```python
from build123d import *

# Parameters (mm, degrees)
F0_W     = 10
F0_H     = 20
F0_W_2   = 5
F1_DEPTH = 2.5


with BuildPart() as f1:
    # F0 (on Front) → F1 (new body, symmetric)
    with BuildSketch(Plane.XZ):
        Polygon((-42.5, -5), (42.5, -5), (42.5, 5), (32.5, 5), (27.5, 5), (22.5, 5), (17.5, 5), (12.5, 5), (7.5, 5), (2.5, 5), (-2.5, 5), (-7.5, 5), (-12.5, 5), (-17.5, 5), (-22.5, 5), (-27.5, 5), (-32.5, 5), (-42.5, 5), align=None)
        with Locations((37.5, 15)):
            Rectangle(F0_W, F0_H)
        with Locations((-37.5, 15)):
            Rectangle(F0_W, F0_H)
        with Locations((25, 15)):
            Rectangle(F0_W_2, F0_H)
        with Locations((-25, 15)):
            Rectangle(F0_W_2, F0_H)
        with Locations((15, 15)):
            Rectangle(F0_W_2, F0_H)
        with Locations((-15, 15)):
            Rectangle(F0_W_2, F0_H)
        with Locations((5, 15)):
            Rectangle(F0_W_2, F0_H)
        with Locations((-5, 15)):
            Rectangle(F0_W_2, F0_H)
    extrude(amount=F1_DEPTH, both=True)


solid = f1.part
```
Geometry: final body of the model. Coordinates: model frame, mm. A direction names the side the tool comes from. Round coordinates to 2 decimals unless told otherwise and drop trailing zeros. Loops run counter-clockwise (first coordinate to the right, second up) from the corner with the lowest first, then second, coordinate; pieces in that order, holes last. Notation, with made-up numbers: (23, -16) -> (59, -16) arc R20 ccw to (59, 12) -> close; hole circle Ø7 at (31, -33). An arc over 180 degrees is marked (long way). Write each question's results on one line, items separated by ' | '.
Item 1: Pull-direction query (X, two-part tool) for faces 1 (the face through (-42.5, 0, 10)), 2 (the face through (-1, -2.5, 4)), 3 (the face through (-27.5, 0, 15)); classes: pulls with the +X half, pulls with the -X half, needs draft (parallel to the pull), parting line crosses it, or undercut.
Answers below:
face 1: pulls with the -X half | face 2: needs draft | face 3: undercut
Item 2: Pin query (flat end, axial travel): pin 1 Ø5 at (x, z) = (-29, 7) entering from +Y; pin 2 Ø2 at (x, y) = (-20, -1.5) entering from +Z. Return the tip coordinate at first contact, or that it passes through.
Answers below:
pin 1: stops at y = 2.5 | pin 2: stops at z = 5
Item 3: Set-up query: faces 4 (the face through (-20, 0, 5)), 5 (the face through (-1, 2.5, 4)). Return all of +Z, -Z, +X, -X, +Y, -Y with unobstructed straight access to the full face (end or side cutting, diameter ignored); none if empty.
Answers below:
face 4: +Z, +Y, -Y | face 5: +Z, -Z, +X, -X, +Y
Item 4: Cut plane C-C on x = 1.5. Return the cut outline in (y, z).
Answers below:
outline: (-2.5, -5) -> (2.5, -5) -> (2.5, 5) -> (-2.5, 5) -> close
Item 5: Line query: probe 1 along Z at (x, y) = (-11.5, -1.5). Output: solid intervals per line, ascending. Write a range as [from, to].
Answers below:
probe 1: z = [-5, 5]
Item 6: Cut plane A-A on z = 15.75. State how many separate pieces and enclosed holes the cut face has, and give its area (3 significant figures).
Answers below:
separate pieces: 8 | enclosed holes: 0 | area: 250 mm²
